Work out the finished part from the listing and answer in its coordinate system (mm). Coordinates: 2 decimals unless noted, no trailing zeros. Loops run counter-clockwise (first coordinate to the right, second up) from the corner with the lowest first, then second, coordinate; pieces in that order, holes last. Notation, with made-up numbers: (29.25, 86) -> (58.25, 86) arc R18 ccw to (58.25, 100) -> close; hole circle Ø2 at (34.5, 1.5). An arc over 180 degrees is marked (long way). Use a Markdown table: item, result. Add a question column.
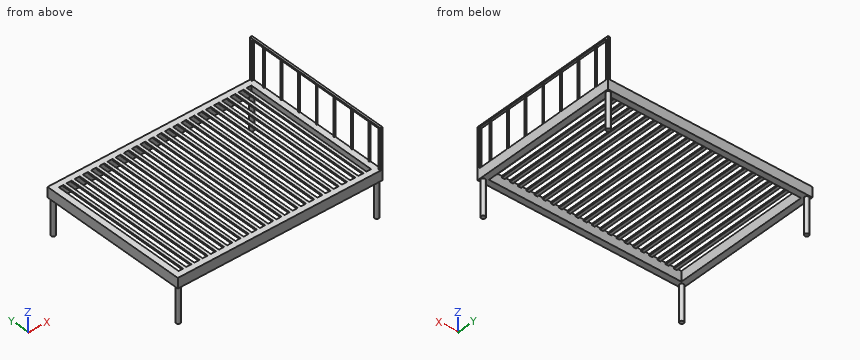
```python
from build123d import *

# Parameters (mm, degrees)
F0_W     = 2023
F0_H     = 1480
F0_W_2   = 30
F0_H_2   = 1360
F1_DEPTH = 15
F2_DEPTH = 100
F3_R     = 20
F4_DEPTH = 350
F5_W     = 20
F5_H     = 20
F5_W_2   = 10
F5_H_2   = 10
F6_DEPTH = 400
F7_W     = 20
F7_H     = 15
F8_DEPTH = 1480


with BuildPart() as f1:
    # F0 (on Top) → F1 (new body)
    with BuildSketch(Plane.XY):
        Rectangle(F0_W, F0_H)
        Polygon((-951.5, -680), (-951.5, 680), (-906.5, 680), (-876.5, 680), (-825.5, 680), (-795.5, 680), (-744.5, 680), (-714.5, 680), (-663.5, 680), (-633.5, 680), (-582.5, 680), (-552.5, 680), (-501.5, 680), (-471.5, 680), (-420.5, 680), (-390.5, 680), (-339.5, 680), (-309.5, 680), (-258.5, 680), (-228.5, 680), (-177.5, 680), (-147.5, 680), (-96.5, 680), (-66.5, 680), (-15.5, 680), (14.5, 680), (65.5, 680), (95.5, 680), (146.5, 680), (176.5, 680), (227.5, 680), (257.5, 680), (308.5, 680), (338.5, 680), (389.5, 680), (419.5, 680), (470.5, 680), (500.5, 680), (551.5, 680), (581.5, 680), (632.5, 680), (662.5, 680), (713.5, 680), (743.5, 680), (794.5, 680), (824.5, 680), (875.5, 680), (905.5, 680), (951.5, 680), (951.5, -680), (905.5, -680), (875.5, -680), (824.5, -680), (794.5, -680), (743.5, -680), (713.5, -680), (662.5, -680), (632.5, -680), (581.5, -680), (551.5, -680), (500.5, -680), (470.5, -680), (419.5, -680), (389.5, -680), (338.5, -680), (308.5, -680), (257.5, -680), (227.5, -680), (176.5, -680), (146.5, -680), (95.5, -680), (65.5, -680), (14.5, -680), (-15.5, -680), (-66.5, -680), (-96.5, -680), (-147.5, -680), (-177.5, -680), (-228.5, -680), (-258.5, -680), (-309.5, -680), (-339.5, -680), (-390.5, -680), (-420.5, -680), (-471.5, -680), (-501.5, -680), (-552.5, -680), (-582.5, -680), (-633.5, -680), (-663.5, -680), (-714.5, -680), (-744.5, -680), (-795.5, -680), (-825.5, -680), (-876.5, -680), (-906.5, -680), align=None, mode=Mode.SUBTRACT)
        with Locations((-891.5, 0)):
            Rectangle(F0_W_2, F0_H_2)
        with Locations((-810.5, 0)):
            Rectangle(F0_W_2, F0_H_2)
        with Locations((-729.5, 0)):
            Rectangle(F0_W_2, F0_H_2)
        with Locations((-648.5, 0)):
            Rectangle(F0_W_2, F0_H_2)
        with Locations((-567.5, 0)):
            Rectangle(F0_W_2, F0_H_2)
        with Locations((-486.5, 0)):
            Rectangle(F0_W_2, F0_H_2)
        with Locations((-405.5, 0)):
            Rectangle(F0_W_2, F0_H_2)
        with Locations((-324.5, 0)):
            Rectangle(F0_W_2, F0_H_2)
        with Locations((-243.5, 0)):
            Rectangle(F0_W_2, F0_H_2)
        with Locations((-162.5, 0)):
            Rectangle(F0_W_2, F0_H_2)
        with Locations((-81.5, 0)):
            Rectangle(F0_W_2, F0_H_2)
        with Locations((-0.5, 0)):
            Rectangle(F0_W_2, F0_H_2)
        with Locations((80.5, 0)):
            Rectangle(F0_W_2, F0_H_2)
        with Locations((161.5, 0)):
            Rectangle(F0_W_2, F0_H_2)
        with Locations((242.5, 0)):
            Rectangle(F0_W_2, F0_H_2)
        with Locations((323.5, 0)):
            Rectangle(F0_W_2, F0_H_2)
        with Locations((404.5, 0)):
            Rectangle(F0_W_2, F0_H_2)
        with Locations((485.5, 0)):
            Rectangle(F0_W_2, F0_H_2)
        with Locations((566.5, 0)):
            Rectangle(F0_W_2, F0_H_2)
        with Locations((647.5, 0)):
            Rectangle(F0_W_2, F0_H_2)
        with Locations((728.5, 0)):
            Rectangle(F0_W_2, F0_H_2)
        with Locations((809.5, 0)):
            Rectangle(F0_W_2, F0_H_2)
        with Locations((890.5, 0)):
            Rectangle(F0_W_2, F0_H_2)
    extrude(amount=-F1_DEPTH)

    # F0 (on Top) → F2 (join)
    with BuildSketch(Plane.XY):
        Rectangle(F0_W, F0_H)
        Polygon((-951.5, -680), (-951.5, 680), (-906.5, 680), (-876.5, 680), (-825.5, 680), (-795.5, 680), (-744.5, 680), (-714.5, 680), (-663.5, 680), (-633.5, 680), (-582.5, 680), (-552.5, 680), (-501.5, 680), (-471.5, 680), (-420.5, 680), (-390.5, 680), (-339.5, 680), (-309.5, 680), (-258.5, 680), (-228.5, 680), (-177.5, 680), (-147.5, 680), (-96.5, 680), (-66.5, 680), (-15.5, 680), (14.5, 680), (65.5, 680), (95.5, 680), (146.5, 680), (176.5, 680), (227.5, 680), (257.5, 680), (308.5, 680), (338.5, 680), (389.5, 680), (419.5, 680), (470.5, 680), (500.5, 680), (551.5, 680), (581.5, 680), (632.5, 680), (662.5, 680), (713.5, 680), (743.5, 680), (794.5, 680), (824.5, 680), (875.5, 680), (905.5, 680), (951.5, 680), (951.5, -680), (905.5, -680), (875.5, -680), (824.5, -680), (794.5, -680), (743.5, -680), (713.5, -680), (662.5, -680), (632.5, -680), (581.5, -680), (551.5, -680), (500.5, -680), (470.5, -680), (419.5, -680), (389.5, -680), (338.5, -680), (308.5, -680), (257.5, -680), (227.5, -680), (176.5, -680), (146.5, -680), (95.5, -680), (65.5, -680), (14.5, -680), (-15.5, -680), (-66.5, -680), (-96.5, -680), (-147.5, -680), (-177.5, -680), (-228.5, -680), (-258.5, -680), (-309.5, -680), (-339.5, -680), (-390.5, -680), (-420.5, -680), (-471.5, -680), (-501.5, -680), (-552.5, -680), (-582.5, -680), (-633.5, -680), (-663.5, -680), (-714.5, -680), (-744.5, -680), (-795.5, -680), (-825.5, -680), (-876.5, -680), (-906.5, -680), align=None, mode=Mode.SUBTRACT)
    extrude(amount=-F2_DEPTH)

    # F3 (on face) → F4 (join)
    with BuildSketch(Plane(origin=(0, 0, -100), x_dir=(1, 0, 0), z_dir=(0, 0, -1))):
        with Locations((-981.5, 710)):
            Circle(F3_R)
        with Locations((981.5, 710)):
            Circle(F3_R)
        with Locations((981.5, -710)):
            Circle(F3_R)
        with Locations((-981.5, -710)):
            Circle(F3_R)
    extrude(amount=F4_DEPTH)

    # F5 (on face) → F6 (join)
    with BuildSketch(Plane.XY):
        with Locations((1001.5, 730)):
            Rectangle(F5_W, F5_H)
        with Locations((1001.5, -730)):
            Rectangle(F5_W, F5_H)
        with Locations((1006.5, -600)):
            Rectangle(F5_W_2, F5_H_2)
        with Locations((1006.5, -400)):
            Rectangle(F5_W_2, F5_H_2)
        with Locations((1006.5, -200)):
            Rectangle(F5_W_2, F5_H_2)
        with Locations((1006.5, 0)):
            Rectangle(F5_W_2, F5_H_2)
        with Locations((1006.5, 200)):
            Rectangle(F5_W_2, F5_H_2)
        with Locations((1006.5, 400)):
            Rectangle(F5_W_2, F5_H_2)
        with Locations((1006.5, 600)):
            Rectangle(F5_W_2, F5_H_2)
    extrude(amount=F6_DEPTH)

    # F7 (on face) → F8 (join, through all)
    with BuildSketch(Plane.XZ.offset(740)):
        with Locations((1001.5, 392.5)):
            Rectangle(F7_W, F7_H)
    extrude(amount=-F8_DEPTH)


solid = f1.part
```
Item 1: Given pin 1 (24 mm diameter, centred on x = 563, y = -58, fed in from -Z); pin 2 (6 mm diameter, centred on x = -736, y = -488.5, fed in from +Z), each flat-ended and moving along its own axis, determine where each tip first touches the part or whether it passes through.
Item 2: Find the intervals of material crossed by probe 1 along X at (y, z) = (473.5, -24); probe 2 along Z at (x, y) = (-258, 405.5), in increasing order.
Item 3: Section A-A (z = -275.5) is taken. Determine the outline of the cut face in (x, y), then the cut area to 3 significant figures.
Item 4: Section B-B (y = 491.5) is taken. Count the separate pieces of the cut face and the enclosed holes in it, then the cut area to 4 significant figures.
Output:
| question | item | result |
|---|---|---|
| 1 | pin 1 | stops at z = -15 |
| 1 | pin 2 | stops at z = 0 |
| 2 | probe 1 | x = -1011.5 to -951.5, 951.5 to 1011.5 |
| 2 | probe 2 | z = -15 to 0 |
| 3 | outline | circle Ø40 at (-981.5, -710); circle Ø40 at (-981.5, 710); circle Ø40 at (981.5, -710); circle Ø40 at (981.5, 710) |
| 3 | area | 5,030 mm2 |
| 4 | separate pieces | 26 |
| 4 | enclosed holes | 0 |
| 4 | area | 22,650 mm2 |
